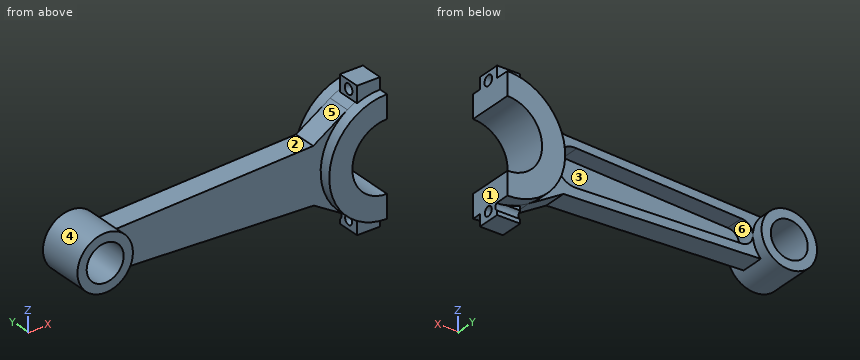
```python
from build123d import *
from build123d.topology import SkipClean

# Parameters (mm, degrees)
EXTRUDE_START       = 5
EXTRUDE_2_DEPTH     = 10
EXTRUDE_4_DEPTH     = 2
EXTRUDE_START_2     = -11
EXTRUDE_5_DEPTH     = 10
EXTRUDE_6_DEPTH     = 20
SKETCH_1_10_R       = 12
EXTRUDE_7_DEPTH     = 10
SKETCH_1_11_R       = 12
EXTRUDE_8_DEPTH     = 20
SKETCH_1_12_R       = 8
CUT_EXTRUDE_1_DEPTH = 20
SKETCH_5_R          = 2
CUT_EXTRUDE_2_DEPTH = 20
EXTRUDE_9_DEPTH     = 20
SKETCH_6_R          = 2.01846984
SKETCH_6_R_2        = 2.203549483
CUT_EXTRUDE_3_DEPTH = 20


with BuildPart() as part:
    # 스케치1 → 보스-돌출2 (new body)
    with BuildSketch(Plane(origin=(0, 0, 0), x_dir=(1, 0, 0), z_dir=(0, 1, 0)).offset(EXTRUDE_START)):
        with BuildLine():
            Line((49.549845173, -12.099230676), (64.355035733, -21.515007377))
            ThreePointArc((64.355035733, -21.515007377), (70.784736297, -24.42375035), (77.771133503, -25.41978705))
            Line((77.771133503, -25.41978705), (77.771133503, -15.41978705))
            ThreePointArc((77.771133503, -15.41978705), (62.771133503, -0.41978705), (77.771133503, 14.58021295))
            Line((77.771133503, 14.58021295), (77.771133503, 24.58021295))
            ThreePointArc((77.771133503, 24.58021295), (71.05915641, 23.662350801), (64.840032894, 20.97616203))
            Line((64.840032894, 20.97616203), (49.823782841, 11.900769324))
            Line((49.823782841, 11.900769324), (-44.228051971, 7.900769324))
            ThreePointArc((-44.228051971, 7.900769324), (-36.228051971, -0.099230676), (-44.228051971, -8.099230676))
            Line((-44.228051971, -8.099230676), (49.549845173, -12.099230676))
        make_face()
        with BuildLine():
            ThreePointArc((44.198484097, 7.559691169), (52.770591505, -0.512908915), (44.012885893, -8.383772269))
            Line((44.012885893, -8.383772269), (-27.228341583, -5))
            ThreePointArc((-27.228341583, -5), (-32.228341583, 0), (-27.228341583, 5))
            Line((-27.228341583, 5), (44.198484097, 7.559691169))
        make_face(mode=Mode.SUBTRACT)
    extrude(amount=EXTRUDE_2_DEPTH)

    # 스케치1<8> → 보스-돌출4 (add)
    with BuildSketch(Plane(origin=(0, 0, 0), x_dir=(1, 0, 0), z_dir=(0, 1, 0)).offset(EXTRUDE_START)):
        with BuildLine():
            Line((44.198484097, 7.559691169), (-27.228341583, 5))
            ThreePointArc((-27.228341583, 5), (-30.774179158, 3.525200121), (-32.228256402, -0.029185644))
            ThreePointArc((-32.228256402, -0.029185644), (-30.753541703, -3.545837575), (-27.228341583, -5))
            Line((-27.228341583, -5), (44.012885893, -8.383772269))
            Line((44.012885893, -8.383772269), (44.771133503, -8.41978705))
            ThreePointArc((44.771133503, -8.41978705), (50.42798774, -6.076641312), (52.771133503, -0.419787086))
            ThreePointArc((52.771133503, -0.419787086), (50.427987765, 5.237067187), (44.771133503, 7.58021295))
            Line((44.771133503, 7.58021295), (44.198484097, 7.559691169))
        make_face()
    extrude(amount=EXTRUDE_4_DEPTH)

    # 스케치2 → 보스-돌출5 (add)
    with BuildSketch(Plane(origin=(0, 15, 0), x_dir=(1, 0, 0), z_dir=(0, 1, 0)).offset(EXTRUDE_START_2)):
        with BuildLine():
            Line((67.771133503, -30.41978705), (77.771133503, -30.41978705))
            Line((77.771133503, -30.41978705), (77.771133503, -25.41978705))
            ThreePointArc((77.771133503, -25.41978705), (72.663392411, -24.892444873), (67.771133503, -23.332665525))
            Line((67.771133503, -23.332665525), (67.771133503, -30.41978705))
        make_face()
        with BuildLine():
            Line((67.771133503, 29.58021295), (67.771133503, 22.493091425))
            ThreePointArc((67.771133503, 22.493091425), (72.663392411, 24.052870773), (77.771133503, 24.58021295))
            Line((77.771133503, 24.58021295), (77.771133503, 29.58021295))
            Line((77.771133503, 29.58021295), (67.771133503, 29.58021295))
        make_face()
    extrude(amount=EXTRUDE_5_DEPTH)

    # 스케치1<9> → 보스-돌출6 (add)
    with BuildSketch(Plane(origin=(0, 0, 0), x_dir=(1, 0, 0), z_dir=(0, 1, 0))):
        with BuildLine():
            Line((-44.228051971, 7.900769324), (-35.625030381, 8.266653588))
            ThreePointArc((-35.625030381, 8.266653588), (-56.22805195, -0.098514915), (-35.626028438, -8.466141165))
            Line((-35.626028438, -8.466141165), (-44.228051971, -8.099230676))
            ThreePointArc((-44.228051971, -8.099230676), (-52.228051971, -0.099230676), (-44.228051971, 7.900769324))
        make_face()
    extrude(amount=EXTRUDE_6_DEPTH)

    # 스케치1<10> → 보스-돌출7 (add)
    with BuildSketch(Plane(origin=(0, 0, 0), x_dir=(1, 0, 0), z_dir=(0, 1, 0))):
        with Locations(Location((-44.228051971, -0.099230676, 0), (0, 0, 44.199354179))):
            Circle(SKETCH_1_10_R)
    extrude(amount=EXTRUDE_7_DEPTH)

    # 스케치1<11> → 보스-돌출8 (add)
    with SkipClean():  # the faces are left unmerged after this step: merging them gives an invalid solid
        with BuildSketch(Plane(origin=(0, 0, 0), x_dir=(1, 0, 0), z_dir=(0, 1, 0))):
            with Locations(Location((-44.228051971, -0.099230676, 0), (0, 0, 270))):
                Circle(SKETCH_1_11_R)
        extrude(amount=EXTRUDE_8_DEPTH)
    add(part.part.scale(1), mode=Mode.REPLACE)  # the faces are merged on a copy

    # 스케치1<12> → 컷-돌출1 (cut)
    with BuildSketch(Plane(origin=(0, 0, 0), x_dir=(1, 0, 0), z_dir=(0, 1, 0))):
        with Locations(Location((-44.228051971, -0.099230676, 0), (0, 0, 90))):
            Circle(SKETCH_1_12_R)
    extrude(amount=CUT_EXTRUDE_1_DEPTH, mode=Mode.SUBTRACT)

    # 스케치5 → 컷-돌출2 (cut)
    with BuildSketch(Plane.ZY.offset(-67.771133503)):
        with Locations((-26.036652187, 15)):
            Circle(SKETCH_5_R)
    extrude(amount=-CUT_EXTRUDE_2_DEPTH, mode=Mode.SUBTRACT)

    # 스케치1<13> → 보스-돌출9 (add)
    with SkipClean():  # the faces are left unmerged after this step: merging them gives an invalid solid
        with BuildSketch(Plane(origin=(0, 0, 0), x_dir=(1, 0, 0), z_dir=(0, 1, 0))):
            with BuildLine():
                Line((77.771133503, 24.58021295), (77.771133503, 14.58021295))
                ThreePointArc((77.771133503, 14.58021295), (62.771133503, -0.41978705), (77.771133503, -15.41978705))
                Line((77.771133503, -15.41978705), (77.771133503, -25.41978705))
                ThreePointArc((77.771133503, -25.41978705), (52.771133503, -0.41978705), (77.771133503, 24.58021295))
            make_face()
        extrude(amount=EXTRUDE_9_DEPTH)
    add(part.part.scale(1), mode=Mode.REPLACE)  # the faces are merged on a copy

    # 스케치6 → 컷-돌출3 (cut)
    with BuildSketch(Plane.ZY.offset(-67.771133503)):
        with Locations((-25.686179168, 8.874314897)):
            Circle(SKETCH_6_R)
        with Locations((26.79403668, 8.874314897)):
            Circle(SKETCH_6_R_2)
    extrude(amount=-CUT_EXTRUDE_3_DEPTH, mode=Mode.SUBTRACT)


solid = part.part
```
Check sheet for the modelled part. Datum: model origin and axes. Units: mm. Face numbers are marked on the shaded views. A direction names the side the tool comes from. Give positions to 0.01 mm unless a question says otherwise; leave off trailing zeros. Write each loop counter-clockwise with the first axis right and the second up, starting at its lowest first coordinate (ties: lowest second). Pieces come first, ordered by that corner, then holes.
Item 1: Cross-section at D-D (x = 38). Enter the section's corners in (y, z).
Item 2: Access from +Z, -Z, +X, -X, +Y, -Y to the whole of each face (thin tool, end or side, straight path). Record for the marked faces 1, 2 and 3.
Item 3: Cross-section at B-B (x = 60). Enter the section's corners in (y, z).
Item 4: Cross-section at C-C (x = -2.5). Enter the section's corners in (y, z), and give its area (3 significant figures).
Item 5: Cross-section at A-A (y = 18.5). Enter the section's corners in (x, z).
Item 6: Gauge pin test, flat ends, axial feed: pin 1 (10.5 mm diameter, centred on x = 37, z = 13.5, fed in from +Y); pin 2 (5.5 mm diameter, centred on y = 8.87, z = 26.79, fed in from +X); pin 3 (13 mm diameter, centred on x = 44.77, z = 0.42, fed in from -Y); pin 4 (3 mm diameter, centred on y = 11, z = -19, fed in from -X). Record the tip position at first contact, or that the pin passes through.
Item 7: Draft check along Z on the marked faces 4, 5 and 6. Enter one of: released by +Z, released by -Z, zero draft, split by the parting line, or undercut.
Item 8: Scan lines: L1, parallel to X at y = 14.5, z = 4; L2, parallel to X at y = 7.5, z = -0.5; L3, parallel to Y at x = -20, z = 2. Record each from-to range of solid material in increasing order.
Report:
1. outline: (5, -11.4) - (15, -11.4) - (15, -7.34) - (7, -7.34) - (7, 8.1) - (15, 8.1) - (15, 11.61) - (5, 11.61) - close
2. face 1: +Z, -Z, +X, +Y, -Y
2. face 2: +Z, +Y, -Y
2. face 3: +Y
3. outline: (0, -17.16) - (5, -17.16) - (5, -18.05) - (15, -18.05) - (15, -17.16) - (20, -17.16) - (20, 18) - (15, 18) - (15, 18.75) - (5, 18.75) - (5, 18) - (0, 18) - close
4. outline: (5, -9.68) - (15, -9.68) - (15, -5.89) - (7, -5.89) - (7, 6.17) - (15, 6.17) - (15, 9.88) - (5, 9.88) - close
4. area: 99.1 mm2
5. outline: circle Ø24 at (-44.23, 0.1); (77.77, -24.58) - (77.77, -14.58) arc R15 cw to (77.77, 15.42) - (77.77, 25.42) arc R25 ccw to start; hole circle Ø16 at (-44.23, 0.1)
6. pin 1: stops at y = 15
6. pin 2: stops at x = 77.77
6. pin 3: stops at y = 5
6. pin 4: stops at x = 59.09
7. face 4: split by the parting line
7. face 5: released by +Z
7. face 6: undercut
8. L1: x = -55.58 to -51.21, -37.24 to -30.23, 51.93 to 63.2
8. L2: x = -56.21 to -52.21, -36.25 to -32.2, 52.72 to 62.8
8. L3: y = 5 to 7
